from build123d import *

# Parameters (mm, degrees)
SKETCH2_R          = 6.604
CUT_EXTRUDE1_DEPTH = 12.7
FILLET1_R          = 6.604
CHAMFER1_SIZE      = 33.02
CHAMFER1_SIZE2     = 23.120852912


with BuildPart() as part:
    # Sketch1 → Revolve1 (revolve)
    with BuildSketch(Plane.XY, mode=Mode.PRIVATE) as revolve1_sk:
        Polygon((0, 51.054), (0, 10.16), (31.75, 10.16), (31.75, 29.943780472), (12.7, 57.15), (-6.35, 57.15), (-6.35, 51.054), align=None)
    revolve(revolve1_sk.sketch.rotate(Axis((0, 0, 0), (1, 0, 0)), 90), axis=Axis((0, 0, 0), (1, 0, 0)))

    # Sketch2 → Cut-Extrude1 (cut)
    with BuildSketch(Plane(origin=(31.75, 0, 0), x_dir=(0, 0, -1), z_dir=(1, 0, 0))):
        with Locations((-19.05, 0)):
            Circle(SKETCH2_R)
        with Locations((0, 19.05)):
            Circle(SKETCH2_R)
        with Locations((19.05, 0)):
            Circle(SKETCH2_R)
        with Locations((0, -19.05)):
            Circle(SKETCH2_R)
    extrude(amount=-CUT_EXTRUDE1_DEPTH, mode=Mode.SUBTRACT)

    # Fillet1
    fillet1_edges = [part.edges().sort_by_distance(p)[0] for p in [
        (19.05, 0, 25.654),
        (19.05, 19.05, 6.604),
        (19.05, 0, -12.446),
        (19.05, -19.05, 6.604),
    ]]
    fillet(fillet1_edges, radius=FILLET1_R)

    # Chamfer1
    chamfer1_edges = [part.edges().sort_by_distance(p)[0] for p in [
        (0, 0, -10.16),
    ]]
    chamfer1_side = [part.faces().sort_by_distance(p)[0] for p in [
        (0, 0, -49.609974816),
    ]]
    chamfer(chamfer1_edges, length=CHAMFER1_SIZE, length2=CHAMFER1_SIZE2, reference=chamfer1_side[0])


solid = part.part
Part model, mm, in its own coordinate system. A direction names the side the tool comes from. Give positions to 0.01 mm unless a question says otherwise; leave off trailing zeros. Loops run counter-clockwise (first coordinate to the right, second up) from the corner with the lowest first, then second, coordinate; pieces in that order, holes last.
(1) Band-saw the part on B-B (x = 6.5). Write the cut outline in (y, z), and give its area (3 significant figures).
Return value:
outline: circle Ø114.3 at (0, 0); hole circle Ø67.79 at (0, 0)
area: 6,650 mm2
(2) Pull direction Y, two halves, no side cores. Call faces 4 (the cylindrical face through (28.745, -12.502, 0.86)), 5 (the flat face through (31.75, 6, -13)), 6 (the cylindrical face through (27.496, -10.074, -1.323)), 7 (the cylindrical face through (3.042, -2.513, -57.095)): pulls with the +Y half, pulls with the -Y half, needs draft (parallel to the pull), parting line crosses it, or undercut.
Return value:
face 4: undercut
face 5: needs draft
face 6: undercut
face 7: parting line crosses it
(3) 3-axis set-ups, long thin cutter, end or side, ignore diameter. For faces 1 (the cylindrical face through (28.745, 0.29, -12.452)), 2 (the flat face through (0, -12, -42)), 3 (the flat face through (-6.35, -47, -21)): which of +Z, -Z, +X, -X, +Y, -Y reach the whole face in a straight line?
Return value:
face 1: +X
face 2: -X
face 3: +Z, -Z, -X, +Y, -Y
(4) Band-saw the part on A-A (x = 28). Write the cut outline in (y, z), and give its area (3 significant figures).
Return value:
outline: circle Ø70.6 at (0, 0); hole circle Ø13.21 at (-19.05, 0); hole circle Ø20.32 at (0, 0); hole circle Ø13.21 at (0, -19.05); hole circle Ø13.21 at (0, 19.05); hole circle Ø13.21 at (19.05, 0)
area: 3,040 mm2
(5) Drill centre lines: line 1 along Y through (x, z) = (-4.5, 0); line 2 along Y through (x, z) = (29, 0); line 3 along Y through (x, z) = (3, 19.5). Where is each one in solid material? Low to high.
Return value:
line 1: y = -57.15 to -51.05, 51.05 to 57.15
line 2: y = -33.87 to -25.65, -12.45 to -10.16, 10.16 to 12.45, 25.65 to 33.87
line 3: y = -53.72 to -33.65, 33.65 to 53.72
(6) Pin check, flat tips, straight feed: pin 1 (3 mm diameter, centred on x = 6.5, z = 44.5, fed in from +Y); pin 2 (4 mm diameter, centred on y = -38, z = -30, fed in from +X); pin 3 (15 mm diameter, centred on y = 0, z = -19.05, fed in from -X). Stop position of each tip, or through.
Return value:
pin 1: stops at y = 37.64
pin 2: stops at x = 20.22
pin 3: stops at x = 11.64
